from build123d import *

# Parameters (mm, degrees)
POCKET_DEPTH       = 145.459123
POCKET_DEPTH_BACK  = 177.459123
POLARPATTERN_COUNT = 5


with BuildPart() as part:
    # Sketch009 → Revolution (revolve)
    with BuildSketch(Plane.YZ):
        with BuildLine():
            Line((-32, 25), (-31.006334, 25))
            Line((-31.006334, 24), (-31.006334, 25))
            Line((-28, 24), (-31.006334, 24))
            Line((-28, 24), (-28, 25))
            Line((-28, 25), (-27, 25))
            Line((-27, 25), (-27, 24))
            Line((-24, 24), (-27, 24))
            Line((-24, 24), (-24, 25))
            Line((-24, 25), (-23, 25))
            Line((-23, 25), (-23, 24))
            Line((-20, 24), (-23, 24))
            Line((-20, 24), (-20, 25))
            Line((-20, 25), (-19, 25))
            Line((-19, 25), (-19, 24))
            Line((-15.98482, 24), (-19, 24))
            Line((-15.98482, 25), (-15.98482, 24))
            Line((-15.98482, 25), (-14.98482, 25))
            Line((-14.98482, 25), (-14.98482, 21.997654))
            ThreePointArc((-15.998639, 21.00955), (-15.282862, 21.289299), (-14.98482, 21.997654))
            Line((-15.998639, 21.00955), (-25.00382, 21.00955))
            ThreePointArc((-25.00382, 21.00955), (-25.68626, 20.700427), (-25.977919, 20.010342))
            Line((-25.977919, 2.4), (-25.977919, 20.010342))
            Line((-28.777919, 2.4), (-25.977919, 2.4))
            Line((-28.777919, 0.8), (-28.777919, 2.4))
            Line((-30.377919, 0.8), (-28.777919, 0.8))
            Line((-30.377919, 1.7), (-30.377919, 0.8))
            Line((-32, 1.7), (-30.377919, 1.7))
            Line((-32, 25), (-32, 1.7))
        make_face()
    revolve(axis=Axis((0, 0, 0), (0, 1, 0)))

    # Sketch010 → Pocket (cut, two sides)
    with BuildSketch(Plane(origin=(-5.2, 0, 0), x_dir=(1, 0, 0), z_dir=(0, -1, 0))) as pocket_sk:
        with BuildLine():
            add(Edge.make_bspline(
                [(11.995053, 15.000581), (5.131915, -6.987182), (-1.338915, 15.000254)],
                knots=[-6.684799, -6.684799, -6.684799, 6.648635, 6.648635, 6.648635], degree=2))
            ThreePointArc((-1.338915, 15.000254), (5.328035, 16.380749), (11.995053, 15.000581))
        make_face()
    pocket = extrude(amount=-POCKET_DEPTH, mode=Mode.SUBTRACT) + extrude(pocket_sk.sketch, amount=POCKET_DEPTH_BACK, mode=Mode.SUBTRACT)

    # PolarPattern: Pocket ×5 about axis
    polarpattern_axis = Axis((0, 0, 0), (0, 1, 0))
    for i in range(1, POLARPATTERN_COUNT):
        add(pocket.rotate(polarpattern_axis, i * 360 / POLARPATTERN_COUNT), mode=Mode.SUBTRACT)


solid = part.part
Geometry: final body of the model. Coordinates: model frame, mm. A direction names the side the tool comes from. Give positions to 0.01 mm unless a question says otherwise; leave off trailing zeros. Put each result on its own line as item: value. Start each with the question number.
1) Ray query, line 1 along Y through (x, z) = (13.5, 20); line 2 along X through (y, z) = (-30.95, 0); line 3 along X through (y, z) = (-19.5, 0). Return the intervals inside material, ascending.
2) Contact query for flat-ended pins moving along their axis: pin 1 (1 mm diameter, centred on x = 0, z = 0, fed in from +Y); pin 2 (8 mm diameter, centred on y = -24, z = 14, fed in from +X); pin 3 (20 mm diameter, centred on x = 4.5, z = -3.5, fed in from +Y); pin 4 (8 mm diameter, centred on x = 12.5, y = -28, fed in from -Z). Output: stop coordinate, or through.
3) Access query for faces 4 (the flat face through (0, -30.378, 1)), 5 (the cylindrical face through (1.055, -21.521, -23.977)), 6 (the cylindrical face through (-15.57, -29.03, 5.09)). Directions: +Z, -Z, +X, -X, +Y, -Y. A direction counts if a zero-diameter tool reaches every point of the face in a straight line with its end or side. Return the directions, or none.
4) Pull-direction query (Y, two-part tool) for faces 1 (the flat face through (22.3, -28, 9.4)), 2 (the cylindrical face through (-9.7, -29, -13.2)), 3 (the flat face through (-4, -25.978, 0)); classes: pulls with the +Y half, pulls with the -Y half, needs draft (parallel to the pull), parting line crosses it, or undercut.
5) Cut plane A-A (z = -12.5). Give the number of separate pieces and of enclosed holes in the cut face, then the cut area to 3 significant figures.
Verdict:
1. line 1: -32 to -31.01, -28 to -27, -24 to -23, -20 to -19, -15.98 to -14.98
1. line 2: -24 to -16.36, -4.82 to -1.7, 1.7 to 4.75, 16.44 to 24
1. line 3: -25 to -21.01, 21.01 to 25
2. pin 1: through
2. pin 2: x = 22.91
2. pin 3: y = -25.98
2. pin 4: z = -23.51
3. face 4: -Y
3. face 5: none
3. face 6: +Y, -Y
4. face 1: undercut
4. face 2: needs draft
4. face 3: pulls with the +Y half
5. separate pieces: 3
5. enclosed holes: 0
5. area: 238 mm2
